Verification items for the finished model (mm, model axes). Face numbers are marked on the shaded views. A direction names the side the tool comes from. Coordinates: 2 decimals unless noted, no trailing zeros. Order: outer loops, then holes, each group sorted by start corner. A loop starts at its lowest first (then second) coordinate and runs counter-clockwise, first axis right, second up. Notation, with made-up numbers: (87, 87) -> (112, 87) arc R24 ccw to (112, 125) -> close; hole circle Ø9 at (65, -23). An arc over 180 degrees is marked (long way). Answer as CSV lines item,"result".
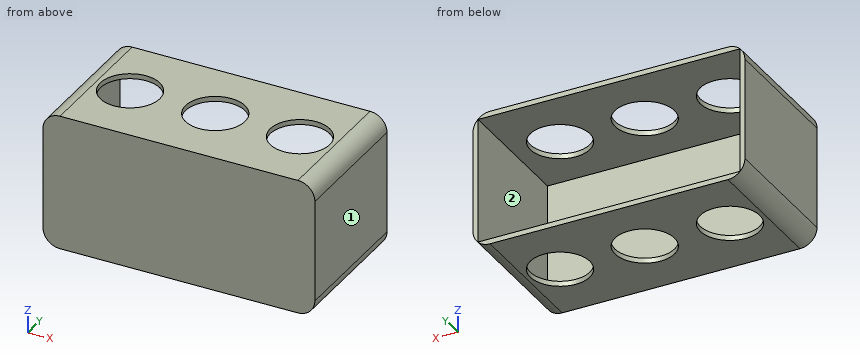
```python
from build123d import *

# Parameters (mm, degrees)
SKETCH1_W           = 160
SKETCH1_H           = 80
BOSS_EXTRUDE1_DEPTH = 80
SHELL1_T            = -3
SKETCH2_R           = 17.5
CUT_EXTRUDE1_DEPTH  = 80
FILLET1_R           = 10


with BuildPart() as part:
    # Sketch1 → Boss-Extrude1 (new body)
    with BuildSketch(Plane(origin=(0, 0, 0), x_dir=(1, 0, 0), z_dir=(0, 1, 0))):
        Rectangle(SKETCH1_W, SKETCH1_H)
    extrude(amount=BOSS_EXTRUDE1_DEPTH)

    # Shell1
    shell1_openings = [part.faces().sort_by_distance(p)[0] for p in [
        (0, 80, 0),
    ]]
    offset(amount=SHELL1_T, openings=shell1_openings, kind=Kind.INTERSECTION)

    # Sketch2 → Cut-Extrude1 (cut)
    with BuildSketch(Plane.XY.offset(40)):
        with Locations((-50, 40)):
            Circle(SKETCH2_R)
        with Locations((0, 40.255057562)):
            Circle(SKETCH2_R)
        with Locations((50, 40)):
            Circle(SKETCH2_R)
    extrude(amount=-CUT_EXTRUDE1_DEPTH, mode=Mode.SUBTRACT)

    # Fillet1
    fillet1_edges = [part.edges().sort_by_distance(p)[0] for p in [
        (80, 40, 40),
        (-80, 40, 40),
        (-80, 40, -40),
        (80, 40, -40),
    ]]
    fillet(fillet1_edges, radius=FILLET1_R)


solid = part.part
```
Item 1: Section check C-C, the plane z = 25. Record the boundary of the cut face in (x, y), plus the area to 3 significant figures.
Answer list:
outline,"(-80, 0) -> (80, 0) -> (80, 80) -> (77, 80) -> (77, 3) -> (-77, 3) -> (-77, 80) -> (-80, 80) -> close"
area,"942 mm2"
Item 2: Thickness scan on line 1 (X direction, y = 50, z = 18); line 2 (Z direction, x = -57, y = 71); line 3 (Y direction, x = 50, z = -37.9). Record the ranges inside material, lowest first.
Answer list:
line 1,"-80 to -77, 77 to 80"
line 2,"-40 to -37, 37 to 40"
line 3,"0 to 22.5, 57.5 to 80"
Item 3: Tool access check on the marked faces 1 and 2. Record the directions out of +Z, -Z, +X, -X, +Y, -Y that give a thin tool (end or side, any length) a straight path to the whole face; none if there is none.
Answer list:
face 1,"+Z, -Z, +X, +Y, -Y"
face 2,"+Y"
Item 4: Section check B-B, the plane y = 18. Record the boundary of the cut face in (x, z).
Answer list:
outline,"(-80, -30) arc R10 ccw to (-70, -40) -> (70, -40) arc R10 ccw to (80, -30) -> (80, 30) arc R10 ccw to (70, 40) -> (-70, 40) arc R10 ccw to (-80, 30) -> close; hole (-77, -37) -> (77, -37) -> (77, 37) -> (-77, 37) -> close"
Item 5: Section check D-D, the plane x = -7. Record the boundary of the cut face in (y, z).
Answer list:
outline,"(0, -40) -> (24.22, -40) -> (24.22, -37) -> (3, -37) -> (3, 37) -> (24.22, 37) -> (24.22, 40) -> (0, 40) -> close; (56.29, -40) -> (80, -40) -> (80, -37) -> (56.29, -37) -> close; (56.29, 37) -> (80, 37) -> (80, 40) -> (56.29, 40) -> close"
Item 6: Section check A-A, the plane x = -50. Record the boundary of the cut face in (y, z).
Answer list:
outline,"(0, -40) -> (22.5, -40) -> (22.5, -37) -> (3, -37) -> (3, 37) -> (22.5, 37) -> (22.5, 40) -> (0, 40) -> close; (57.5, -40) -> (80, -40) -> (80, -37) -> (57.5, -37) -> close; (57.5, 37) -> (80, 37) -> (80, 40) -> (57.5, 40) -> close"
